Verification items for the finished model (mm, model axes). Face numbers are marked on the shaded views. Give positions to 0.01 mm unless a question says otherwise; leave off trailing zeros. Write each loop counter-clockwise with the first axis right and the second up, starting at its lowest first coordinate (ties: lowest second). Pieces come first, ordered by that corner, then holes. Notation, with made-up numbers: (44, 41) - (101, 41) arc R21 cw to (101, 62) - close; hole circle Ø1 at (76, -8.75). An arc over 180 degrees is marked (long way). Answer as a JSON object with one key per item and string values. Group by question number.
Item 1: Scan lines: line 1 along X through (y, z) = (83, 17.75); line 2 along Y through (x, z) = (58, 7.5); line 3 along X through (y, z) = (-18, 18.5). Record each from-to range of solid material in increasing order. Write a range as [from, to].
Item 2: Sectioned sample at A-A, the plane x = -84. Record the boundary of the cut face in (y, z), and give its area (3 significant figures).
Item 3: Sectioned sample at C-C, the plane x = 164.5. Record the boundary of the cut face in (y, z), and give its area (3 significant figures).
Item 4: Sectioned sample at B-B, the plane z = 6.5. Count the separate pieces of the cut face and the enclosed holes in it, and give its area (3 significant figures).
Item 5: Go/stop test with flat-tipped pins: pin 1 (10 mm diameter, centred on y = -31, z = 8, fed in from -X); pin 2 (6 mm diameter, centred on x = -14.65, y = -26.78, fed in from -Z); pin 3 (6 mm diameter, centred on x = -65.5, y = 93, fed in from -Z). Record where each tip stops, or that it passes through.
Item 6: Draft check along Y on the marked faces 1, 2 and 3. Enter one of: +Y half, -Y half, draft (parallel to the pull), parting line (faces both ways), or undercut.
```python
from build123d import *

# Parameters (mm, degrees)
SKETCH_1_R          = 23.5
EXTRUDE_1_DEPTH     = 20
SKETCH_2_R          = 2.5
CUT_EXTRUDE_1_DEPTH = 290.447601331
SKETCH_5_R          = 2.5
CUT_EXTRUDE_3_DEPTH = 290.447601331
SKETCH_6_R          = 9.5
SKETCH_6_R_2        = 1.5
CUT_EXTRUDE_4_DEPTH = 290.447601331
FILLET_1_R          = 5
FILLET_2_R          = 5
FILLET_3_R          = 5
FILLET_4_R          = 5
FILLET_5_R          = 15
FILLET_6_R          = 15


with BuildPart() as part:
    # 草图1 → 凸台-拉伸1 (new body)
    with BuildSketch(Plane.XY):
        Polygon((-112.146066939, 163.723609917), (237.853933061, 163.723609917), (237.853933061, -6.276390083), (107.853933061, -6.276390083), (107.853933061, -54.276390083), (-32.146066939, -54.276390083), (-32.146066939, -6.276390083), (-112.146066939, -6.276390083), align=None)
        with Locations((177.853933061, 73.723609917)):
            Circle(SKETCH_1_R, mode=Mode.SUBTRACT)
        with Locations((-67.146066939, 73.723609917)):
            Circle(SKETCH_1_R, mode=Mode.SUBTRACT)
    extrude(amount=EXTRUDE_1_DEPTH)

    # 草图2 → 切除-拉伸1 (cut, through all)
    with BuildSketch(Plane.XY.offset(20)):
        with Locations((47.853933061, -34.276390083)):
            Circle(SKETCH_2_R)
        with Locations((57.853933061, -46.276390083)):
            Circle(SKETCH_2_R)
    extrude(amount=-CUT_EXTRUDE_1_DEPTH, mode=Mode.SUBTRACT)

    # 草图5 → 切除-拉伸3 (cut, through all)
    with BuildSketch(Plane.XY.offset(20)):
        with Locations((-24.646066939, -16.776390083)):
            Circle(SKETCH_5_R)
        with Locations((-14.646066939, -26.776390083)):
            Circle(SKETCH_5_R)
    extrude(amount=-CUT_EXTRUDE_3_DEPTH, mode=Mode.SUBTRACT)

    # 草图6 → 切除-拉伸4 (cut, through all)
    with BuildSketch(Plane.XY.offset(20)):
        with Locations((86.853933061, -33.276390083)):
            Circle(SKETCH_6_R)
        with Locations((71.353933061, -17.776390083)):
            Circle(SKETCH_6_R_2)
        with Locations(Location((71.353933061, -48.776390083, 0), (0, 0, 180))):
            Circle(SKETCH_6_R_2)
        with Locations((102.353933061, -48.776390083)):
            Circle(SKETCH_6_R_2)
        with Locations(Location((102.353933061, -17.776390083, 0), (0, 0, 180))):
            Circle(SKETCH_6_R_2)
    extrude(amount=-CUT_EXTRUDE_4_DEPTH, mode=Mode.SUBTRACT)

    # 圆角1
    fillet_1_edges = [part.edges().sort_by_distance(p)[0] for p in [
        (-32.146066939, -54.276390083, 10),
    ]]
    fillet(fillet_1_edges, radius=FILLET_1_R)

    # 圆角2
    fillet_2_edges = [part.edges().sort_by_distance(p)[0] for p in [
        (107.853933061, -54.276390083, 10),
    ]]
    fillet(fillet_2_edges, radius=FILLET_2_R)

    # 圆角3
    fillet_3_edges = [part.edges().sort_by_distance(p)[0] for p in [
        (237.853933061, -6.276390083, 10),
    ]]
    fillet(fillet_3_edges, radius=FILLET_3_R)

    # 圆角4
    fillet_4_edges = [part.edges().sort_by_distance(p)[0] for p in [
        (-112.146066939, -6.276390083, 10),
    ]]
    fillet(fillet_4_edges, radius=FILLET_4_R)

    # 圆角5
    fillet_5_edges = [part.edges().sort_by_distance(p)[0] for p in [
        (-112.146066939, 163.723609917, 10),
    ]]
    fillet(fillet_5_edges, radius=FILLET_5_R)

    # 圆角6
    fillet_6_edges = [part.edges().sort_by_distance(p)[0] for p in [
        (237.853933061, 163.723609917, 10),
    ]]
    fillet(fillet_6_edges, radius=FILLET_6_R)


solid = part.part
```
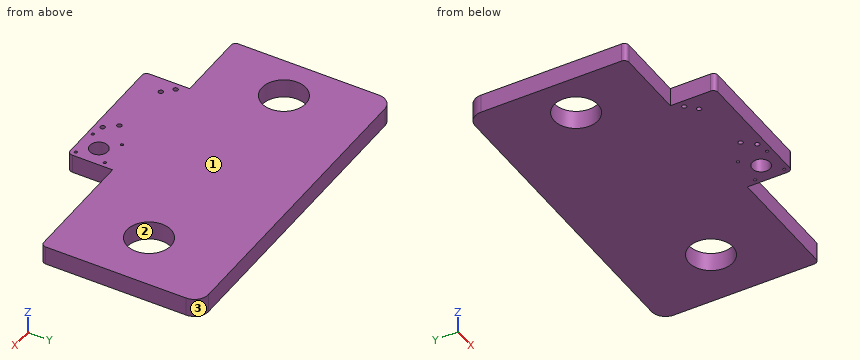
Geometry check:
{
 "1": {"line 1": "[-112.15, -88.74], [-45.55, 156.26], [199.45, 237.85]", "line 2": "[-54.28, -48.77], [-43.78, 163.72]", "line 3": "[-32.15, -26.83], [-22.47, 69.87], [72.84, 100.87], [103.84, 107.85]"},
 "2": {"outline": "(-6.28, 0) - (57.35, 0) - (57.35, 20) - (-6.28, 20) - close; (90.1, 0) - (163.72, 0) - (163.72, 20) - (90.1, 20) - close", "area": "2,740 mm^2"},
 "3": {"outline": "(-6.28, 0) - (54.39, 0) - (54.39, 20) - (-6.28, 20) - close; (93.06, 0) - (163.72, 0) - (163.72, 20) - (93.06, 20) - close", "area": "2,630 mm^2"},
 "4": {"separate pieces": "1", "enclosed holes": "11", "area": "62,200 mm^2"},
 "5": {"pin 1": "x = -32.15", "pin 2": "z = 0", "pin 3": "through"},
 "6": {"face 1": "draft", "face 2": "undercut", "face 3": "+Y half"}
}
